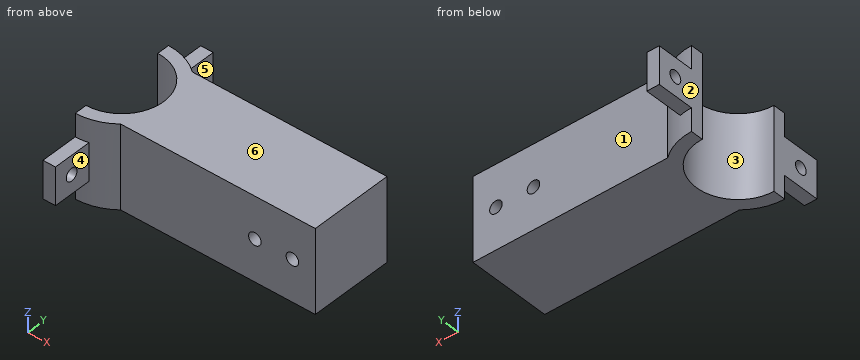
from build123d import *

# Parameters (mm, degrees)
EXTRUDE_1_DEPTH     = 20
SKETCH_2_R          = 1.5
CUT_EXTRUDE_1_DEPTH = 63.880839689
SKETCH_6_R          = 1.5
EXTRUDE_2_DEPTH     = 3


with BuildPart() as part:
    # Эскиз1 → Бобышка-Вытянуть1 (new body)
    with BuildSketch(Plane.XY):
        with BuildLine():
            Line((0, 10), (0, 13))
            ThreePointArc((0, 13), (4.415880433, 12.227019261), (8.306623863, 10))
            Line((8.306623863, 10), (55, 10))
            Line((55, 10), (55, 0))
            Line((55, 0), (55, -10))
            Line((55, -10), (8.306623863, -10))
            ThreePointArc((8.306623863, -10), (4.415880433, -12.227019261), (0, -13))
            Line((0, -13), (0, -10))
            ThreePointArc((0, -10), (10, 0), (0, 10))
        make_face()
    extrude(amount=EXTRUDE_1_DEPTH)

    # Эскиз2 → Вырез-Вытянуть1 (cut, through all)
    with BuildSketch(Plane(origin=(0, 10, 0), x_dir=(1, 0, 0), z_dir=(0, 1, 0))):
        with Locations(Location((40.5, -10, 0), (0, 0, 270))):
            Circle(SKETCH_2_R)
        with Locations(Location((49.5, -10, 0), (0, 0, 270))):
            Circle(SKETCH_2_R)
    extrude(amount=-CUT_EXTRUDE_1_DEPTH, mode=Mode.SUBTRACT)

    # Эскиз6 → Бобышка-Вытянуть2 (add)
    # profile 1 of 2: a face of its own
    with BuildSketch(Plane.ZY):
        Polygon((10, 10), (5.5, 10), (5.5, 22), (14.5, 22), (14.5, 10), align=None)
        with Locations((10, 17.5)):
            Circle(SKETCH_6_R, mode=Mode.SUBTRACT)
    # profile 2 of 2: a face of its own
    with BuildSketch(Plane.ZY):
        Polygon((10, -10), (5.5, -10), (5.5, -22), (14.5, -22), (14.5, -10), align=None)
        with Locations((10, -17.5)):
            Circle(SKETCH_6_R, mode=Mode.SUBTRACT)
    extrude(amount=-EXTRUDE_2_DEPTH)


solid = part.part
For this review, take the finished solid that the model builds, in its own axes (mm). Face numbers are marked on the shaded views. A direction names the side the tool comes from. Coordinates: 2 decimals unless noted, no trailing zeros. Write each loop counter-clockwise with the first axis right and the second up, starting at its lowest first coordinate (ties: lowest second). Pieces come first, ordered by that corner, then holes. Notation, with made-up numbers: (10, 43.25) -> (40, 43.25) arc R31 cw to (40, 77.25) -> close; hole circle Ø8 at (-37.5, 71.25). An arc over 180 degrees is marked (long way). Write each question's results on one line, items separated by ' | '. Start each with the question number.
1) For the marked faces 4, 5 and 6, list the 3-axis set-ups (+Z, -Z, +X, -X, +Y, -Y) from which the entire face can be reached by the end or side of a thin tool; tool diameter is ignored.
2) Consider section D-D (y = 0). Write out the cut boundary in (x, z).
3) Wall thickness on L1, parallel to X at y = 3.25, z = 10; L2, parallel to X at y = -4.5, z = 10.5; L3, parallel to Y at x = 2, z = 10: over which ranges is each line inside the solid? List them lowest first. Write a range as [from, to].
4) Consider section B-B (z = 10). Write out the cut boundary in (x, y).
5) The part is to be moulded in two halves that separate along Y. For the marked faces 1, 2 and 3, say which applies: +Y half, -Y half, draft (parallel to the pull), parting line (faces both ways), or undercut.
6) Insertion check: pin 1 (12 mm diameter, centred on x = 39.5, z = 5.5, fed in from +Y); pin 2 (2.5 mm diameter, centred on y = -17.5, z = 10, fed in from -X); pin 3 (3.5 mm diameter, centred on x = 2, y = -19, fed in from -Z); pin 4 (10 mm diameter, centred on y = 18, z = 9, fed in from +X). Each pin has a flat end and moves straight along its axis. Give the tip position at first contact, or say it passes through.
7) Consider section C-C (y = 17.5). Write out the cut boundary in (x, z).
8) Consider section A-A (x = 49.5). Write out the cut boundary in (y, z).
Geometry says:
1) face 4: +Z, -Z, +X, -Y | face 5: +Z, -Z, +X, +Y | face 6: +Z, +X, -X, +Y, -Y
2) outline: (10, 0) -> (55, 0) -> (55, 20) -> (10, 20) -> close; hole circle Ø3 at (40.5, 10); hole circle Ø3 at (49.5, 10)
3) L1: [9.46, 39], [42, 48], [51, 55] | L2: [8.93, 39.09], [41.91, 48.09], [50.91, 55] | L3: [-22, -19], [-16, -9.8], [9.8, 16], [19, 22]
4) outline: (0, -22) -> (3, -22) -> (3, -19) -> (0, -19) -> close; (0, -16) -> (3, -16) -> (3, -12.65) arc R13 ccw to (8.31, -10) -> (39, -10) -> (39, 10) -> (8.31, 10) arc R13 ccw to (3, 12.65) -> (3, 16) -> (0, 16) -> (0, 10) arc R10 cw to (0, -10) -> close; (0, 19) -> (3, 19) -> (3, 22) -> (0, 22) -> close; (42, -10) -> (48, -10) -> (48, 10) -> (42, 10) -> close; (51, -10) -> (55, -10) -> (55, 10) -> (51, 10) -> close
5) face 1: +Y half | face 2: draft | face 3: undercut
6) pin 1: y = 10 | pin 2: through | pin 3: z = 5.5 | pin 4: x = 3
7) outline: (0, 5.5) -> (3, 5.5) -> (3, 8.5) -> (0, 8.5) -> close; (0, 11.5) -> (3, 11.5) -> (3, 14.5) -> (0, 14.5) -> close
8) outline: (-10, 0) -> (10, 0) -> (10, 8.5) -> (-10, 8.5) -> close; (-10, 11.5) -> (10, 11.5) -> (10, 20) -> (-10, 20) -> close
